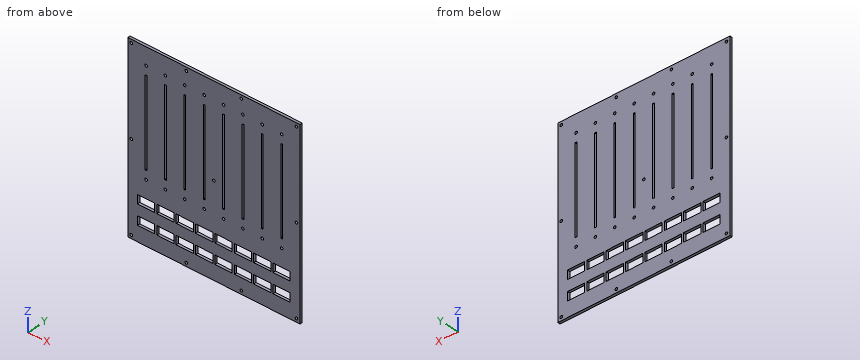
from build123d import *

# Parameters (mm, degrees)
SKETCH1_W                 = 200
SKETCH1_H                 = 210
BOSS_EXTRUDE1_DEPTH       = 3
CUT_EXTRUDE1_REACH        = 147.031
SKETCH2_R                 = 1.5
SKETCH2_W                 = 2
SKETCH2_H                 = 100
LPATTERN1_COUNT           = 8
LPATTERN1_PITCH           = 22.5
CUT_EXTRUDE2_REACH        = 147.031
SKETCH3_W                 = 20
SKETCH3_H                 = 10
LPATTERN2_COUNT           = 8
LPATTERN2_PITCH           = 22.5
LPATTERN2_COUNT_DIR2      = 2
LPATTERN2_PITCH_DIR2      = 22.5
CUT_EXTRUDE3_REACH        = 147.031
SKETCH4_R                 = 1.5
LPATTERN3_COUNT           = 4
LPATTERN3_PITCH           = 64
LPATTERN4_COUNT           = 2
LPATTERN4_PITCH           = 202
LPATTERN4_COPY_1_REACH    = 147.031
LPATTERN4_COPY_1_SKETCH_R = 1.5
LPATTERN4_COPY_2_REACH    = 147.031
LPATTERN4_COPY_2_SKETCH_R = 1.5
LPATTERN4_COPY_3_REACH    = 147.031
LPATTERN4_COPY_3_SKETCH_R = 1.5
CUT_EXTRUDE4_REACH        = 147.031
SKETCH8_R                 = 1.5
CUT_EXTRUDE5_REACH        = 147.031
SKETCH9_R                 = 1.5


with BuildPart() as part:
    # Sketch1 → Boss-Extrude1 (new body)
    with BuildSketch(Plane(origin=(0, 0, 0), x_dir=(1, 0, 0), z_dir=(0, 1, 0))):
        Rectangle(SKETCH1_W, SKETCH1_H)
    extrude(amount=BOSS_EXTRUDE1_DEPTH)

    # Sketch2 → Cut-Extrude1 (cut, up to next)
    with BuildSketch(Plane(origin=(0, 3, 0), x_dir=(1, 0, 0), z_dir=(0, 1, 0)), mode=Mode.PRIVATE) as cut_extrude1_sk1:
        with Locations(Location((-78.75, -85, 0), (0, 0, 270))):
            Circle(SKETCH2_R)
    cut_extrude1_tool1 = extrude(cut_extrude1_sk1.sketch, amount=-CUT_EXTRUDE1_REACH, mode=Mode.PRIVATE) & part.part
    # Sketch2 → Cut-Extrude1 (cut, up to next)
    with BuildSketch(Plane(origin=(0, 3, 0), x_dir=(1, 0, 0), z_dir=(0, 1, 0)), mode=Mode.PRIVATE) as cut_extrude1_sk2:
        with Locations(Location((-78.75, 35, 0), (0, 0, 270))):
            Circle(SKETCH2_R)
    cut_extrude1_tool2 = extrude(cut_extrude1_sk2.sketch, amount=-CUT_EXTRUDE1_REACH, mode=Mode.PRIVATE) & part.part
    # Sketch2 → Cut-Extrude1 (cut, up to next)
    with BuildSketch(Plane(origin=(0, 3, 0), x_dir=(1, 0, 0), z_dir=(0, 1, 0)), mode=Mode.PRIVATE) as cut_extrude1_sk3:
        with Locations((-78.75, -25)):
            Rectangle(SKETCH2_W, SKETCH2_H)
    cut_extrude1_tool3 = extrude(cut_extrude1_sk3.sketch, amount=-CUT_EXTRUDE1_REACH, mode=Mode.PRIVATE) & part.part
    cut_extrude1_1 = cut_extrude1_tool1.solids().sort_by_distance((-78.75, 3, 85))[0]
    add(cut_extrude1_1, mode=Mode.SUBTRACT)
    cut_extrude1_2 = cut_extrude1_tool2.solids().sort_by_distance((-78.75, 3, -35))[0]
    add(cut_extrude1_2, mode=Mode.SUBTRACT)
    cut_extrude1_3 = cut_extrude1_tool3.solids().sort_by_distance((-78.75, 3, 25))[0]
    add(cut_extrude1_3, mode=Mode.SUBTRACT)
    cut_extrude1 = cut_extrude1_1 + cut_extrude1_2 + cut_extrude1_3  # Cut-Extrude1 as one shape, for the pattern or mirror that repeats it

    # LPattern1: Cut-Extrude1 ×8
    with Locations(*[(i * LPATTERN1_PITCH, 0, 0) for i in range(1, LPATTERN1_COUNT)]):
        add(cut_extrude1, mode=Mode.SUBTRACT)

    # Sketch3 → Cut-Extrude2 (cut, up to next)
    with BuildSketch(Plane(origin=(0, 3, 0), x_dir=(1, 0, 0), z_dir=(0, 1, 0)), mode=Mode.PRIVATE) as cut_extrude2_sk1:
        with Locations((-78.75, 60)):
            Rectangle(SKETCH3_W, SKETCH3_H)
    cut_extrude2_tool1 = extrude(cut_extrude2_sk1.sketch, amount=-CUT_EXTRUDE2_REACH, mode=Mode.PRIVATE) & part.part
    cut_extrude2 = cut_extrude2_tool1.solids().sort_by_distance((-78.75, 3, -60))[0]
    add(cut_extrude2, mode=Mode.SUBTRACT)

    # LPattern2: Cut-Extrude2 8 × 2
    with Locations(*[(i * LPATTERN2_PITCH, 0, -j * LPATTERN2_PITCH_DIR2) for i in range(LPATTERN2_COUNT) for j in range(LPATTERN2_COUNT_DIR2) if (i, j) != (0, 0)]):
        add(cut_extrude2, mode=Mode.SUBTRACT)

    # Sketch4 → Cut-Extrude3 (cut, up to next)
    with BuildSketch(Plane(origin=(0, 3, 0), x_dir=(1, 0, 0), z_dir=(0, 1, 0)), mode=Mode.PRIVATE) as cut_extrude3_sk1:
        with Locations(Location((-96, 101, 0), (0, 0, 270))):
            Circle(SKETCH4_R)
    cut_extrude3_tool1 = extrude(cut_extrude3_sk1.sketch, amount=-CUT_EXTRUDE3_REACH, mode=Mode.PRIVATE) & part.part
    cut_extrude3 = cut_extrude3_tool1.solids().sort_by_distance((-96, 3, -101))[0]
    add(cut_extrude3, mode=Mode.SUBTRACT)

    # LPattern3: Cut-Extrude3 ×4
    with Locations(*[(i * LPATTERN3_PITCH, 0, 0) for i in range(1, LPATTERN3_COUNT)]):
        add(cut_extrude3, mode=Mode.SUBTRACT)

    # LPattern4: Cut-Extrude3 ×2
    with Locations(*[(0, 0, i * LPATTERN4_PITCH) for i in range(1, LPATTERN4_COUNT)]):
        add(cut_extrude3, mode=Mode.SUBTRACT)

    # LPattern4 copy 1 sketch → LPattern4 copy 1 (cut, up to next)
    with BuildSketch(Plane(origin=(64, 3, 202), x_dir=(1, 0, 0), z_dir=(0, 1, 0)), mode=Mode.PRIVATE) as lpattern4_copy_1_sk1:
        with Locations(Location((-96, 101, 0), (0, 0, 270))):
            Circle(LPATTERN4_COPY_1_SKETCH_R)
    lpattern4_copy_1_tool1 = extrude(lpattern4_copy_1_sk1.sketch, amount=-LPATTERN4_COPY_1_REACH, mode=Mode.PRIVATE) & part.part
    add(lpattern4_copy_1_tool1.solids().sort_by_distance((-32, 3, 101))[0], mode=Mode.SUBTRACT)

    # LPattern4 copy 2 sketch → LPattern4 copy 2 (cut, up to next)
    with BuildSketch(Plane(origin=(128, 3, 202), x_dir=(1, 0, 0), z_dir=(0, 1, 0)), mode=Mode.PRIVATE) as lpattern4_copy_2_sk1:
        with Locations(Location((-96, 101, 0), (0, 0, 270))):
            Circle(LPATTERN4_COPY_2_SKETCH_R)
    lpattern4_copy_2_tool1 = extrude(lpattern4_copy_2_sk1.sketch, amount=-LPATTERN4_COPY_2_REACH, mode=Mode.PRIVATE) & part.part
    add(lpattern4_copy_2_tool1.solids().sort_by_distance((32, 3, 101))[0], mode=Mode.SUBTRACT)

    # LPattern4 copy 3 sketch → LPattern4 copy 3 (cut, up to next)
    with BuildSketch(Plane(origin=(192, 3, 202), x_dir=(1, 0, 0), z_dir=(0, 1, 0)), mode=Mode.PRIVATE) as lpattern4_copy_3_sk1:
        with Locations(Location((-96, 101, 0), (0, 0, 270))):
            Circle(LPATTERN4_COPY_3_SKETCH_R)
    lpattern4_copy_3_tool1 = extrude(lpattern4_copy_3_sk1.sketch, amount=-LPATTERN4_COPY_3_REACH, mode=Mode.PRIVATE) & part.part
    add(lpattern4_copy_3_tool1.solids().sort_by_distance((96, 3, 101))[0], mode=Mode.SUBTRACT)

    # Sketch8 → Cut-Extrude4 (cut, up to next)
    with BuildSketch(Plane(origin=(0, 3, 0), x_dir=(1, 0, 0), z_dir=(0, 1, 0)), mode=Mode.PRIVATE) as cut_extrude4_sk1:
        with Locations(Location((0, 0, 0), (0, 0, 270))):
            Circle(SKETCH8_R)
    cut_extrude4_tool1 = extrude(cut_extrude4_sk1.sketch, amount=-CUT_EXTRUDE4_REACH, mode=Mode.PRIVATE) & part.part
    add(cut_extrude4_tool1.solids().sort_by_distance((0, 3, 0))[0], mode=Mode.SUBTRACT)

    # Sketch9 → Cut-Extrude5 (cut, up to next)
    with BuildSketch(Plane(origin=(0, 3, 0), x_dir=(1, 0, 0), z_dir=(0, 1, 0)), mode=Mode.PRIVATE) as cut_extrude5_sk1:
        with Locations(Location((-96, 0, 0), (0, 0, 270))):
            Circle(SKETCH9_R)
    cut_extrude5_tool1 = extrude(cut_extrude5_sk1.sketch, amount=-CUT_EXTRUDE5_REACH, mode=Mode.PRIVATE) & part.part
    # Sketch9 → Cut-Extrude5 (cut, up to next)
    with BuildSketch(Plane(origin=(0, 3, 0), x_dir=(1, 0, 0), z_dir=(0, 1, 0)), mode=Mode.PRIVATE) as cut_extrude5_sk2:
        with Locations(Location((96, 0, 0), (0, 0, 270))):
            Circle(SKETCH9_R)
    cut_extrude5_tool2 = extrude(cut_extrude5_sk2.sketch, amount=-CUT_EXTRUDE5_REACH, mode=Mode.PRIVATE) & part.part
    add(cut_extrude5_tool1.solids().sort_by_distance((-96, 3, 0))[0], mode=Mode.SUBTRACT)
    add(cut_extrude5_tool2.solids().sort_by_distance((96, 3, 0))[0], mode=Mode.SUBTRACT)


solid = part.part
Work out the finished part from the listing and answer in its coordinate system (mm). Give positions to 0.01 mm unless a question says otherwise; leave off trailing zeros. Loops run counter-clockwise (first coordinate to the right, second up) from the corner with the lowest first, then second, coordinate; pieces in that order, holes last. Notation, with made-up numbers: (27.25, 5) -> (76.25, 5) arc R18 ccw to (76.25, 22) -> close; hole circle Ø9 at (56.25, -23). An arc over 180 degrees is marked (long way). Use a Markdown table: item, result. Add a question column.
1. Section A-A on x = -63 is taken. Determine the outline of the cut face in (y, z).
2. Section B-B on z = -8 is taken. State how many separate pieces and enclosed holes the cut face has, and give its area (3 significant figures).
3. Find the intervals of material crossed by probe 1 along Z at (x, y) = (-11.25, 1.05); probe 2 along Z at (x, y) = (-96, 0.85); probe 3 along Z at (x, y) = (-73, 2.3), in increasing order.
4. A flat-ended cylindrical pin translates along its axis: pin 1 Ø2.5 at (x, z) = (11.25, -35) entering from +Y. Find the tip coordinate at first contact, or state that the pin passes through.
Results below:
| question | item | result |
|---|---|---|
| 1 | outline | (0, -105) -> (3, -105) -> (3, -87.5) -> (0, -87.5) -> close; (0, -77.5) -> (3, -77.5) -> (3, -65) -> (0, -65) -> close; (0, -55) -> (3, -55) -> (3, 105) -> (0, 105) -> close |
| 2 | separate pieces | 9 |
| 2 | enclosed holes | 0 |
| 2 | area | 552 mm^2 |
| 3 | probe 1 | z = -105 to -87.5, -77.5 to -65, -55 to -36.5, -33.5 to -25, 75 to 83.5, 86.5 to 105 |
| 3 | probe 2 | z = -105 to -102.5, -99.5 to -1.5, 1.5 to 99.5, 102.5 to 105 |
| 3 | probe 3 | z = -105 to -87.5, -77.5 to -65, -55 to 105 |
| 4 | pin 1 | passes through |
